Part model, mm, in its own coordinate system. Face numbers are marked on the shaded views. A direction names the side the tool comes from. Give positions to 0.01 mm unless a question says otherwise; leave off trailing zeros. Write each loop counter-clockwise with the first axis right and the second up, starting at its lowest first coordinate (ties: lowest second). Pieces come first, ordered by that corner, then holes.
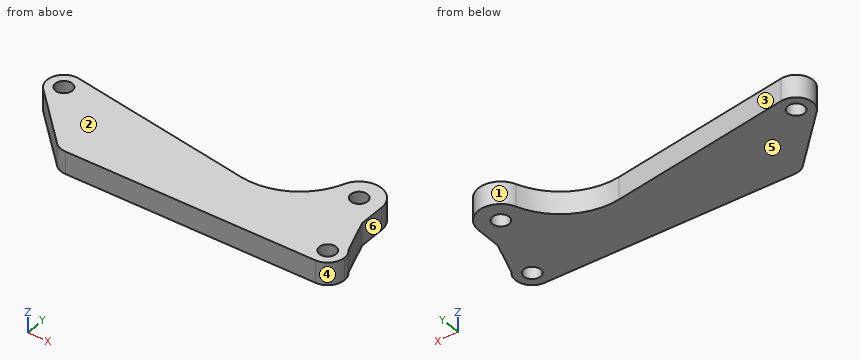
from build123d import *

# Parameters (mm, degrees)
SKETCH1_R           = 1.5
BOSS_EXTRUDE1_DEPTH = 4
FILLET3_R           = 3
CHAMFER1_DEPTH      = 4


with BuildPart() as part:
    # Sketch1 → Boss-Extrude1 (new body)
    with BuildSketch(Plane.XY):
        with BuildLine():
            Line((0, 0), (48.899957301, 0))
            Line((48.899957301, 0), (48.899957301, 6))
            Line((48.899957301, 6), (45.899957301, 6))
            Line((45.899957301, 6), (45.899957301, 16))
            ThreePointArc((45.899957301, 16), (42.622776894, 19.934149442), (38.161191383, 17.42184015))
            ThreePointArc((38.161191383, 17.42184015), (33.02844755, 11.405508249), (25.246040765, 10))
            Line((25.246040765, 10), (-7.780505141, 15.473258612))
            ThreePointArc((-7.780505141, 15.473258612), (-10.939117439, 13.885145013), (-10.392304845, 10.392304845))
            Line((-10.392304845, 10.392304845), (0, 0))
        make_face()
        with Locations((41.899957301, 16)):
            Circle(SKETCH1_R, mode=Mode.SUBTRACT)
        with Locations((-8.270984502, 12.513625189)):
            Circle(SKETCH1_R, mode=Mode.SUBTRACT)
        with Locations((45.899957301, 3)):
            Circle(SKETCH1_R, mode=Mode.SUBTRACT)
    extrude(amount=BOSS_EXTRUDE1_DEPTH)

    # Fillet3
    fillet3_edges = [part.edges().sort_by_distance(p)[0] for p in [
        (0, 0, 2),
        (48.899957301, 0, 2),
        (48.899957301, 6, 2),
    ]]
    fillet(fillet3_edges, radius=FILLET3_R - 0.0001)  # a hair under: the kernel refuses the full size

    # Chamfer1: read off the stored shape, not the designer's step
    # Chamfer1 outline → Chamfer1 (add)
    with BuildSketch(Plane.XY):
        with BuildLine():
            Line((48.207649608, 4.916913199), (45.899957301, 11.306623863))
            Line((45.899957301, 11.306623863), (45.899957301, 6))
            ThreePointArc((45.899957301, 6), (47.174567124, 5.715763207), (48.207649608, 4.916913199))
        make_face()
    extrude(amount=CHAMFER1_DEPTH)


solid = part.part
1) 3-axis set-ups, long thin cutter, end or side, ignore diameter. For the marked faces 5 and 6: which of +Z, -Z, +X, -X, +Y, -Y reach the whole face in a straight line?
Check result:
face 5: -Z, +X, -X, +Y, -Y
face 6: +Z, -Z, +X, +Y
2) Mould opens along X. For the marked faces 1, 2, 3 and 4 say: +X half, -X half, draft (parallel to the pull), parting line (faces both ways), or undercut.
Check result:
face 1: parting line
face 2: draft
face 3: undercut
face 4: +X half
3) Saw through at D-D (x = 2). Write the cut outline in (y, z), and give its area (3 significant figures).
Check result:
outline: (0, 0) - (13.85, 0) - (13.85, 4) - (0, 4) - close
area: 55.4 mm2
4) Saw through at C-C (x = 12.5). Write the cut outline in (y, z).
Check result:
outline: (0, 0) - (12.11, 0) - (12.11, 4) - (0, 4) - close
5) Saw through at B-B (z = 2.15). State how many separate pieces and enclosed holes the cut face has, and give its area (3 significant figures).
Check result:
separate pieces: 1
enclosed holes: 3
area: 706 mm2
6) Flat gauge pins, fed straight in: P1, Ø1.5, axis at y = 6, z = 2.5, coming from the -X side; P2, Ø1.5, axis at y = 4, z = 1.5, coming from the +X side. Where does each tip first touch, or does it go through?
Check result:
P1: stops at x = -6.75
P2: stops at x = 48.89
7) Saw through at A-A (y = 3.75). Write the cut outline in (x, z).
Check result:
outline: (-3.75, 0) - (44.6, 0) - (44.6, 4) - (-3.75, 4) - close; (47.2, 0) - (48.8, 0) - (48.8, 4) - (47.2, 4) - close
8) Drill centre lines: L1, parallel to Y at x = -7.5, z = 0.7; L2, parallel to Y at x = 7.5, z = 3.05; L3, parallel to Y at x = 43.5, z = 3. Where is each one in solid material? Low to high.
Check result:
L1: y = 7.5 to 11.23, 13.8 to 15.43
L2: y = 0 to 12.94
L3: y = 0 to 19.67
